Autodesk Inventor part; units mm, degrees
ref_plane "YZ Plane" through (0, 0, 0) normal (1, 0, 0) x (0, 1, 0)
ref_plane "XZ Plane" through (0, 0, 0) normal (0, 1, 0) x (-1, 0, 0)
ref_plane "XY Plane" through (0, 0, 0) normal (0, 0, 1) x (1, 0, 0)
sketch "Sketch1" plane through (0, 0, 0) normal (0, 1, 0) x (-1, 0, 0)
  line L0 (0, 0) -> (0, -40)
  line L1 (0, -40) -> (40, -40)
  line L2 (40, -40) -> (40, 0)
  line L3 (40, 0) -> (0, 0)
  line L4 (0, 0) -> (1.5, 0)
  line L5 (1.5, 0) -> (1.5, -40)
  line L6 (1.5, -40) -> (0, -40)
  circle A0 centre (20, -20) radius 13.5
  circle A1 centre (20, -4.25) radius 1.5
  circle A2 centre (33.6399, -12.125) radius 1.5
  circle A3 centre (33.6399, -27.875) radius 1.5
  circle A4 centre (20, -35.75) radius 1.5
  circle A5 centre (6.3601, -27.875) radius 1.5
  circle A6 centre (6.3601, -12.125) radius 1.5
  dimension "d0" = 40
  dimension "d2" = 1.5
  dimension "d7" = 3
  dimension "d8" = 3
  dimension "d9" = 3
  dimension "d10" = 3
  dimension "d11" = 3
  dimension "d12" = 3
extrude "Extrusion1" add sketch "Sketch1" along normal blind 1.5 contours L3 L2 L1 L5
extrude "Extrusion2" add sketch "Sketch1" along normal blind 20 contours L3 L5 L1 L0
sketch "Sketch2" plane through (0, 0, 0) normal (1, 0, 0) x (0, 0, -1)
  line L0 (0, 20) -> (5.5, 20)
  line L1 (0, 20) -> (40, 20)
  line L2 (0, 20) -> (34.5, 20)
  line L3 (40, 20) -> (34.5, 20)
  line L4 (34.5, 20) -> (34.5, 16)
  line L5 (34.5, 16) -> (34.5, 10)
  line L6 (34.5, 10) -> (34.5, 4)
  line L7 (5.5, 20) -> (5.5, 16)
  line L8 (5.5, 16) -> (5.5, 10)
  line L9 (5.5, 10) -> (5.5, 4)
  circle A0 centre (5.5, 4) radius 1.5
  circle A1 centre (5.5, 10) radius 1.5
  circle A2 centre (5.5, 16) radius 1.5
  circle A3 centre (34.5, 16) radius 1.5
  circle A4 centre (34.5, 10) radius 1.5
  circle A5 centre (34.5, 4) radius 1.5
  point P0 (0, 0)
  dimension "d17" = 5.5
  dimension "d18" = 34.5
  dimension "d19" = 4
  dimension "d20" = 6
  dimension "d21" = 6
  dimension "d22" = 4
  dimension "d23" = 6
  dimension "d24" = 6
  dimension "d25" = 3
  dimension "d26" = 3
  dimension "d27" = 3
  dimension "d28" = 3
  dimension "d29" = 3
  dimension "d30" = 3
extrude "Extrusion3" cut sketch "Sketch2" against normal blind 5
fillet "Fillet1" radius 10 2 edges at (-40, 0.75, 0) (-40, 0.75, -40)
properties part number "offcenter_L_clamp"
Source: CAD feature listing. Evaluate the final solid. Frame: model axes, mm. Coordinates: 2 decimals unless noted, no trailing zeros. Loops run counter-clockwise (first coordinate to the right, second up) from the corner with the lowest first, then second, coordinate; pieces in that order, holes last. Notation, with made-up numbers: (1, -34.75) - (38, -34.75) arc R15 ccw to (38, -13.75) - close; hole circle Ø8 at (-18, 54). An arc over 180 degrees is marked (long way). Answer as CSV lines item,"result".
1. Section D-D (x = -7). Return loops of the section in (y, z), then the cut area to 3 significant figures.
Established:
outline,"(0, -40) - (1.5, -40) - (1.5, -29.23) - (0, -29.23) - close; (0, -26.52) - (1.5, -26.52) - (1.5, -23.64) - (0, -23.64) - close; (0, -16.36) - (1.5, -16.36) - (1.5, -13.48) - (0, -13.48) - close; (0, -10.77) - (1.5, -10.77) - (1.5, 0) - (0, 0) - close"
area,"40.9 mm2"
2. Ray query, line 1 (Z direction, x = -20, y = 0.9); line 2 (Z direction, x = -0.9, y = 10); line 3 (Y direction, x = -1.05, z = -5.5). Return the intervals inside material, ascending.
Established:
line 1,"z = -40 to -37.25, -34.25 to -33.5, -6.5 to -5.75, -2.75 to 0"
line 2,"z = -40 to -36, -33 to -7, -4 to 0"
line 3,"y = 0 to 2.5, 5.5 to 8.5, 11.5 to 14.5, 17.5 to 20"
3. Section C-C (z = -35). Return loops of the section in (x, y).
Established:
outline,"(-38.66, 0) - (-21.3, 0) - (-21.3, 1.5) - (-38.66, 1.5) - close; (-18.7, 0) - (0, 0) - (0, 2.59) - (-1.5, 2.59) - (-1.5, 1.5) - (-18.7, 1.5) - close; (-1.5, 5.41) - (0, 5.41) - (0, 8.59) - (-1.5, 8.59) - close; (-1.5, 11.41) - (0, 11.41) - (0, 14.59) - (-1.5, 14.59) - close; (-1.5, 17.41) - (0, 17.41) - (0, 20) - (-1.5, 20) - close"
4. Mould query, pull axis Y, two halves, no side actions, for faces 1 (the flat face through (-6, 0, -20)), 2 (the flat face through (-20, 1.5, -6)), 3 (the cylindrical face through (-0.74, 17.01, -4.39)). Classes: released by +Y, released by -Y, zero draft, split by the parting line, or undercut.
Established:
face 1,"released by -Y"
face 2,"released by +Y"
face 3,"undercut"
5. Contact query for flat-ended pins moving along their axis: pin 1 (2.5 mm diameter, centred on x = -20, z = -35.75, fed in from -Y); pin 2 (4 mm diameter, centred on y = 4, z = -5.5, fed in from +X); pin 3 (5 mm diameter, centred on y = 16, z = -34.5, fed in from -X). Output: stop coordinate, or through.
Established:
pin 1,"passes through"
pin 2,"stops at x = 0"
pin 3,"stops at x = -1.5"
6. Section B-B (z = -20). Return loops of the section in (x, y).
Established:
outline,"(-40, 0) - (-33.5, 0) - (-33.5, 1.5) - (-40, 1.5) - close; (-6.5, 0) - (0, 0) - (0, 20) - (-1.5, 20) - (-1.5, 1.5) - (-6.5, 1.5) - close"
7. Section A-A (y = 10). Return loops of the section in (x, z).
Established:
outline,"(-1.5, -40) - (0, -40) - (0, -36) - (-1.5, -36) - close; (-1.5, -33) - (0, -33) - (0, -7) - (-1.5, -7) - close; (-1.5, -4) - (0, -4) - (0, 0) - (-1.5, 0) - close"
